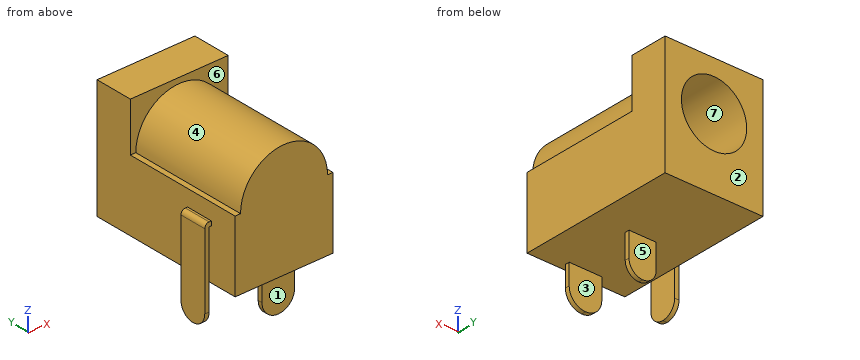
Autodesk Inventor part; units mm, degrees
sketch "スケッチ1" plane through (0, 0, 0) normal (0, 1, 0) x (-1, 0, 0)
  line L0 (-4.5, 11) -> (4.5, 11)
  line L1 (4.5, 11) -> (4.5, 0)
  line L2 (4.5, 0) -> (-4.5, 0)
  line L3 (-4.5, 0) -> (-4.5, 11)
  point P0 (0, 0)
  dimension "d0" = 9
  dimension "d1" = 4.5
  dimension "d2" = 11
extrude "押し出し1" add sketch "スケッチ1" against normal blind 3.5
sketch "スケッチ3" plane through (0, 0, 0) normal (0, 1, 0) x (-1, 0, 0)
  circle A0 centre (0, 6.5) radius 4
  line L0 (-4, 6.5) -> (4, 6.5)
  line L1 (4, 6.5) -> (4, 0)
  line L2 (4, 0) -> (-4, 0)
  line L3 (-4, 0) -> (-4, 6.5)
  point P0 (0, 0)
  dimension "d9" = 8
  dimension "d10" = 6.5
extrude "押し出し3" add sketch "スケッチ3" against normal blind 14.5
ref_plane "作業平面1" through (0, -9.5, 0) normal (0, 1, 0) x (-1, 0, 0)
sketch "スケッチ4" plane through (0, 0, 0) normal (0, 1, 0) x (-1, 0, 0)
  point P0 (0, 0)
sketch "スケッチ5" plane through (0, 0, 0) normal (0, 1, 0) x (-1, 0, 0)
  line L0 (-4.5, 0) -> (4.5, 0)
  line L1 (4.5, 0) -> (4.5, 6.5)
  line L2 (4.5, 6.5) -> (-4.5, 6.5)
  line L3 (-4.5, 6.5) -> (-4.5, 0)
  point P0 (0, 0)
  dimension "d14" = 4.5
  dimension "d15" = 9
  dimension "d16" = 6.5
extrude "押し出し4" add sketch "スケッチ5" against normal blind 14.5
sketch "スケッチ6" plane through (0, -9.5, 0) normal (0, 1, 0) x (-1, 0, 0)
  line L0 (5.1, 5) -> (4.9, 5)
  line L1 (4.9, 5) -> (4.9, -3.5)
  line L2 (4.9, -3.5) -> (5.1, -3.5)
  line L3 (5.1, -3.5) -> (5.1, 5)
  line L4 (0, -13.24) -> (0, 15.04)
  line L5 (4.7, 5) -> (4.9, 5)
  line L6 (4.9, 5) -> (4.9, -3.5)
  line L7 (4.9, -3.5) -> (4.7, -3.5)
  line L8 (4.7, -3.5) -> (4.7, 5)
  line L9 (5.1, 5) -> (0, 5)
  line L10 (0, 5) -> (0, 4.6)
  line L11 (0, 4.6) -> (5.1, 4.6)
  line L12 (5.1, 4.6) -> (5.1, 5)
  point P0 (0, 0)
  dimension "d19" = 4.9
  dimension "d20" = 0.2
  dimension "d21" = 3.5
  dimension "d22" = 5
  dimension "d27" = 0.2
  dimension "d28" = 0.4
extrude "押し出し5" add sketch "スケッチ6" against normal blind 2.5
ref_plane "作業平面2" through (0, -10.75, 0) normal (0, 1, 0) x (-1, 0, 0)
fillet "フィレット1" radius 0.4 1 edges at (-5.1, -10.75, 5)
ref_plane "作業平面4" through (0, -13.7, 0) normal (0, 1, 0) x (-1, 0, 0)
sketch "スケッチ7" plane through (0, -13.7, 0) normal (0, 1, 0) x (-1, 0, 0)
  line L0 (1.5, 5.7) -> (-1.5, 5.7)
  line L1 (-1.5, 5.7) -> (-1.5, -3.4)
  line L2 (-1.5, -3.4) -> (1.5, -3.4)
  line L3 (1.5, -3.4) -> (1.5, 5.7)
  point P0 (0, 0)
  dimension "d31" = 1.5
  dimension "d32" = 3
extrude "押し出し6" add sketch "スケッチ7" along normal mid plane 0.4
fillet "フィレット2" radius 1.5 1 edges at (-1.5, -13.7, -3.4)
fillet "フィレット2" radius 1.5 1 edges at (1.5, -13.7, -3.4)
ref_plane "作業平面5" through (0, -7.7, 0) normal (0, 1, 0) x (-1, 0, 0)
sketch "スケッチ8" plane through (0, -7.7, 0) normal (0, 1, 0) x (-1, 0, 0)
  line L0 (1.25, 6.5) -> (-1.25, 6.5)
  line L1 (-1.25, 6.5) -> (-1.25, -3.5)
  line L2 (-1.25, -3.5) -> (1.25, -3.5)
  line L3 (1.25, -3.5) -> (1.25, 6.5)
  line L4 (4.5, 0) -> (-4.5, 0)
  point P0 (0, 0)
  dimension "d38" = 3.5
  dimension "d39" = 2.5
  dimension "d40" = 1.25
  dimension "d41" = 6.5
extrude "押し出し7" add sketch "スケッチ8" along normal mid plane 0.4
fillet "フィレット3" radius 1.25 1 edges at (1.25, -7.7, -3.5)
fillet "フィレット3" radius 1.25 3 edges at (-1.25, -7.7, -3.5) (-4.9, -9.5, -3.5) (-4.9, -12, -3.5)
sketch "スケッチ9" plane through (0, 0, 0) normal (0, 1, 0) x (-1, 0, 0)
  circle A0 centre (0, 6.5) radius 3
  point P0 (0, 0)
  dimension "d46" = 6
  dimension "d47" = 6.5
extrude "押し出し8" cut sketch "スケッチ9" against normal blind 10
sketch "スケッチ2" plane through (0, 0, 0) normal (0, 1, 0) x (-1, 0, 0)
  circle A0 centre (0, 6.5) radius 3
  line L0 (4.5, 0) -> (-4.5, 0)
  point P0 (0, 0)
  dimension "d5" = 6
  dimension "d6" = 6.5
properties part number "MJ179PH"
The model under review builds one solid part; all positions refer to its coordinate system, in mm. Face numbers are marked on the shaded views. A direction names the side the tool comes from. Round coordinates to 2 decimals unless told otherwise and drop trailing zeros. Loops run counter-clockwise (first coordinate to the right, second up) from the corner with the lowest first, then second, coordinate; pieces in that order, holes last. Notation, with made-up numbers: M -21.5,7.5 L 30.5,7.5 A32 cw 30.5,44.5 Z; hole C 6,16 d7. An arc over 180 degrees is marked long. Put each result on its own line as item: value.
Q1. For pin 1 (3 mm diameter, centred on x = -0.5, z = -2, fed in from +Y); pin 2 (3 mm diameter, centred on x = 0, z = -2, fed in from -Y); pin 3 (5.5 mm diameter, centred on y = -6, z = 3, fed in from -X), all flat-tipped, find the tip position at first contact; note any pin that passes through.
Result set:
pin 1: stops at y = -7.5
pin 2: stops at y = -13.9
pin 3: stops at x = -4.5
Q2. Consider section D-D, the plane z = 9. Give the boundary of the cut face in (x, y).
Result set:
outline: M -4.5,-3.5 L -3.12,-3.5 L -3.12,-14.5 L 3.12,-14.5 L 3.12,-3.5 L 4.5,-3.5 L 4.5,0 L 1.66,0 L 1.66,-10 L -1.66,-10 L -1.66,0 L -4.5,0 Z
Q3. Mouldability with a two-part tool opening along Y and no side actions: class the marked faces 1, 2, 3 and 4 as released by +Y, released by -Y, zero draft, split by the parting line, or undercut.
Result set:
face 1: released by -Y
face 2: released by +Y
face 3: undercut
face 4: zero draft
Q4. Consider section B-B, the plane y = -8.5. Give the boundary of the cut face in (x, z).
Result set:
outline: M -4.5,0 L 4.5,0 L 4.5,6.5 L 4,6.5 A4 ccw -4,6.5 L -4.5,6.5 Z; hole C 0,6.5 d6
Q5. Consider section C-C, the plane x = 4.25. Give the boundary of the cut face in (y, z), then the cut area to 3 significant figures.
Result set:
outline: M -14.5,0 L 0,0 L 0,11 L -3.5,11 L -3.5,6.5 L -14.5,6.5 Z
area: 110 mm²
Q6. To check wall thickness, follow L1, parallel to Z at x = 0, y = -3.75; L2, parallel to Z at x = 0, y = -2.5; L3, parallel to Y at x = -0.75, z = -2. State the ranges of each line that lie inside material, in increasing order.
Result set:
L1: z = 0 to 3.5, 9.5 to 10.5
L2: z = 0 to 3.5, 9.5 to 11
L3: y = -13.9 to -13.5, -7.9 to -7.5
Q7. Machinability: for the marked faces 5, 6 and 7, which of the approach directions +Z, -Z, +X, -X, +Y, -Y give a long, thin tool a straight path to every point of the face, cutting with its end or side? Answer none if there is none.
Result set:
face 5: -Z, +X, -X, +Y
face 6: +Z, -Y
face 7: +Y
Q8. Consider section A-A, the plane z = -1.5. Give the boundary of the cut face in (x, y), then the cut area to 3 significant figures.
Result set:
outline: M -5.1,-12 L -4.7,-12 L -4.7,-9.5 L -5.1,-9.5 Z; M -1.5,-13.9 L 1.5,-13.9 L 1.5,-13.5 L -1.5,-13.5 Z; M -1.25,-7.9 L 1.25,-7.9 L 1.25,-7.5 L -1.25,-7.5 Z
area: 3.20 mm²
